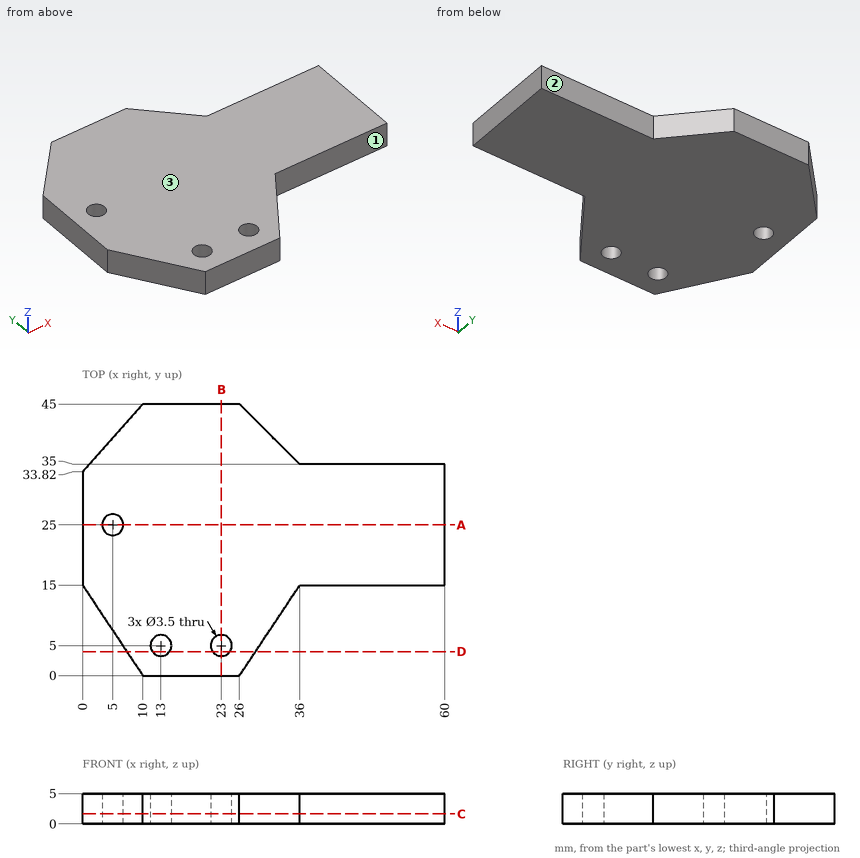
The drawing under review shows one solid part. Ordinate dimensions are in mm from its lowest x, y, z. A direction names the side the tool comes from. Coordinates: 2 decimals unless noted, no trailing zeros. Write each loop counter-clockwise with the first axis right and the second up, starting at its lowest first coordinate (ties: lowest second). Pieces come first, ordered by that corner, then holes. Notation, with made-up numbers: (-5, 38) - (9, 38) arc R12 cw to (9, 54) - close; hole circle Ø2 at (-40, 59). An arc over 180 degrees is marked (long way). Answer as CSV lines item,"result".
(1) We need section C-C (z = 1.65). Give the boundary of the cut face in (x, y), plus the area to 3 significant figures.
Data:
outline,"(0, 15) - (10, 0) - (26, 0) - (36, 15) - (60, 15) - (60, 35) - (36, 35) - (26, 45) - (10, 45) - (0, 33.82) - close; hole circle Ø3.5 at (5, 25); hole circle Ø3.5 at (13, 5); hole circle Ø3.5 at (23, 5)"
area,"1,820 mm2"
(2) Clearance check with flat-ended pins moving along their axes: pin 1 Ø1 at (x, z) = (9, 3.5) entering from -Y; pin 2 Ø3 at (x, y) = (5, 25) entering from -Z. State where each tip first meets the part, or that it passes through.
Data:
pin 1,"stops at y = 0.75"
pin 2,"passes through"
(3) We need section B-B (x = 23). Give the boundary of the cut face in (y, z).
Data:
outline,"(0, 0) - (3.25, 0) - (3.25, 5) - (0, 5) - close; (6.75, 0) - (45, 0) - (45, 5) - (6.75, 5) - close"
(4) For line 1 along X through (y, z) = (4, 1.6) (1 decimal); line 2 along Y through (x, z) = (23, 1.8); line 3 along Y through (x, z) = (12, 2.1) (1 decimal), list the stretches that pass through material, from the lowest coordinate up. Write a range as [from, to].
Data:
line 1,"x = [7.3, 11.6], [14.4, 21.6], [24.4, 28.7]"
line 2,"y = [0, 3.25], [6.75, 45]"
line 3,"y = [0, 3.6], [6.4, 45]"
(5) We need section A-A (y = 25). Give the boundary of the cut face in (x, z).
Data:
outline,"(0, 0) - (3.25, 0) - (3.25, 5) - (0, 5) - close; (6.75, 0) - (60, 0) - (60, 5) - (6.75, 5) - close"
(6) Tool access review of the marked faces 1, 2 and 3: name each direction out of +Z, -Z, +X, -X, +Y, -Y from which nothing blocks a thin tool from reaching the whole face with its end or side.
Data:
face 1,"+Z, -Z, +X, -Y"
face 2,"+Z, -Z, +X, +Y"
face 3,"+Z, +X, -X, +Y, -Y"
(7) We need section D-D (y = 4). Give the boundary of the cut face in (x, z).
Data:
outline,"(7.33, 0) - (11.56, 0) - (11.56, 5) - (7.33, 5) - close; (14.44, 0) - (21.56, 0) - (21.56, 5) - (14.44, 5) - close; (24.44, 0) - (28.67, 0) - (28.67, 5) - (24.44, 5) - close"
